Source: CAD feature listing. Evaluate the final solid. Frame: model axes, mm. A direction names the side the tool comes from. Give positions to 0.01 mm unless a question says otherwise; leave off trailing zeros. Write each loop counter-clockwise with the first axis right and the second up, starting at its lowest first coordinate (ties: lowest second). Pieces come first, ordered by that corner, then holes. Notation, with made-up numbers: (49, 42.25) -> (81, 42.25) arc R12 ccw to (81, 57.25) -> close; hole circle Ø2 at (88.25, 20.5). An arc over 180 degrees is marked (long way). Use one line per item in the form item = value. Start each with the question number.
(1) Material intervals for line 1 along Y through (x, z) = (-19.8, 6.3); line 2 along Y through (x, z) = (13, 10.5); line 3 along X through (y, z) = (9, 3), sorted ascending. Write a range as from..to.
(2) Set-up query: faces 1 (the face through (-24, -1, 11.5)), 2 (the face through (-25, 0, 12)), 3 (the face through (-22.5, 0, 13)). Return all of +Z, -Z, +X, -X, +Y, -Y with unobstructed straight access to the full face (end or side cutting, diameter ignored); none if empty.
(3) First-contact query: P1, Ø0.8, axis at x = -23.5, z = 7, coming from the +Y side (3 decimals); P2, Ø1.8, axis at x = 19.8, y = -14.3, coming from the +Z side; P3, Ø1, axis at y = 2, z = 7, coming from the -X side. Flat tips, straight axial feed; report the tip coordinate or a pass-through.
(4) Cut plane D-D, the plane z = 18.75. Output: boundary loops of the cut face in (x, y), and give its area (3 significant figures).
(5) Cut plane C-C, the plane x = -5. Output: boundary loops of the cut face in (y, z), and give its area (4 significant figures).
(6) Cut plane B-B, the plane y = -1. Output: boundary loops of the cut face in (x, z).
(7) Cut plane A-A, the plane z = 6.5. Count the separate pieces of the cut face and the enclosed holes in it, and give its area (3 significant figures).
(8) Draft query along X for faces 4 (the face through (25, 0, 10)), 5 (the face through (24, 10, 10)), 6 (the face through (20.537, 14.976, 4.965)). Return one class per face: pulls with the +X half, pulls with the -X half, needs draft (parallel to the pull), parting line crosses it, or undercut.
from build123d import *

# Parameters (mm, degrees)
F1_DEPTH        = 20
F2_T            = 2.5
F2_T3_DEPTH     = 25
F3_R            = 2.5
F4_DEPTH        = 5
F11_W           = 3
F11_H           = 2
F12_DEPTH       = 5
F13_DEPTH       = 5
F14_W           = 11
F14_H           = 9
F15_DEPTH       = 5
F16_D           = 2
F16_DEPTH       = 10
F16_TIP         = 0.600860619
F17_D           = 2
F17_DEPTH       = 5
F17_TIP         = 0.600860619
F17_ON_F7_D     = 2
F17_ON_F7_DEPTH = 5
F17_ON_F7_TIP   = 0.600860619
F17_ON_F6_D     = 2
F17_ON_F6_DEPTH = 5
F17_ON_F6_TIP   = 0.600860619
F17_ON_F8_D     = 2
F17_ON_F8_DEPTH = 5
F17_ON_F8_TIP   = 0.600860619


# Not quite as in the source:
# - a shell that OpenCascade refuses in one call is made with other operations: the cavity is built on its own and cut out


with BuildPart() as f1:
    # F0 (on Top) → F1 (new body)
    with BuildSketch(Plane.XY):
        with BuildLine():
            Line((-25, 17.5), (-25, 20))
            Line((-25, 20), (-22.5, 20))
            ThreePointArc((-22.5, 20), (-26.767766953, 21.767766953), (-25, 17.5))
        make_face()
        with BuildLine():
            Line((-22.5, 20), (-25, 20))
            Line((-25, 20), (-25, 17.5))
            ThreePointArc((-25, 17.5), (-23.232233047, 18.232233047), (-22.5, 20))
        make_face()
        with BuildLine():
            Line((22.5, 20), (-22.5, 20))
            ThreePointArc((-22.5, 20), (-23.232233047, 18.232233047), (-25, 17.5))
            Line((-25, 17.5), (-25, -17.5))
            ThreePointArc((-25, -17.5), (-23.232233047, -18.232233047), (-22.5, -20))
            Line((-22.5, -20), (22.5, -20))
            ThreePointArc((22.5, -20), (23.232233047, -18.232233047), (25, -17.5))
            Line((25, -17.5), (25, 17.5))
            ThreePointArc((25, 17.5), (23.232233047, 18.232233047), (22.5, 20))
        make_face()
        with BuildLine():
            ThreePointArc((27.5, 20), (25, 22.5), (22.5, 20))
            Line((22.5, 20), (25, 20))
            Line((25, 20), (25, 17.5))
            ThreePointArc((25, 17.5), (26.767766953, 18.232233047), (27.5, 20))
        make_face()
        with BuildLine():
            Line((25, 20), (22.5, 20))
            ThreePointArc((22.5, 20), (23.232233047, 18.232233047), (25, 17.5))
            Line((25, 17.5), (25, 20))
        make_face()
        with BuildLine():
            ThreePointArc((-22.5, -20), (-23.232233047, -18.232233047), (-25, -17.5))
            Line((-25, -17.5), (-25, -20))
            Line((-25, -20), (-22.5, -20))
        make_face()
        with BuildLine():
            Line((-25, -20), (-25, -17.5))
            ThreePointArc((-25, -17.5), (-26.767766953, -21.767766953), (-22.5, -20))
            Line((-22.5, -20), (-25, -20))
        make_face()
        with BuildLine():
            ThreePointArc((27.5, -20), (26.767766953, -18.232233047), (25, -17.5))
            Line((25, -17.5), (25, -20))
            Line((25, -20), (22.5, -20))
            ThreePointArc((22.5, -20), (25, -22.5), (27.5, -20))
        make_face()
        with BuildLine():
            Line((25, -20), (25, -17.5))
            ThreePointArc((25, -17.5), (23.232233047, -18.232233047), (22.5, -20))
            Line((22.5, -20), (25, -20))
        make_face()
    extrude(amount=F1_DEPTH)

    # F2: shell of thickness 2.5, made by hand


with BuildPart() as f2_core1:
    # F2_t2: copy of F1
    add(f1.part)

    # the walls: a layer under each face that stays
    f2_faces = [f2_core1.faces().sort_by_distance(p)[0] for p in [
        (-25, 0, 10),
        (0, -20, 10),
        (25, 0, 10),
        (0, 20, 10),
        (0, 0, 0),
    ]]
    thicken(f2_faces, amount=-F2_T, mode=Mode.SUBTRACT)

    # F2_s4 → F2_t3 (cut)
    with BuildSketch(Plane.XY.offset(-2.5)):
        Polygon((-22.475, 20.025), (-25, 20), (-25, 17.5), (-22.5, 17.5), align=None)
        Polygon((-25.025, 17.475), (-25, 20), (-22.5, 20), (-22.5, 17.5), align=None)
        Polygon((-25.025, -17.475), (-22.5, -17.5), (-22.5, -20), (-25, -20), align=None)
        Polygon((-22.475, -20.025), (-25, -20), (-25, -17.5), (-22.5, -17.5), align=None)
        Polygon((22.475, -20.025), (22.5, -17.5), (25, -17.5), (25, -20), align=None)
        Polygon((25.025, -17.475), (25, -20), (22.5, -20), (22.5, -17.5), align=None)
        Polygon((25.025, 17.475), (22.5, 17.5), (22.5, 20), (25, 20), align=None)
        Polygon((22.475, 20.025), (25, 20), (25, 17.5), (22.5, 17.5), align=None)
    extrude(amount=F2_T3_DEPTH, mode=Mode.SUBTRACT)


with BuildPart() as f1_1:
    add(f1.part)

    # what is left inside the walls is the cavity
    f2_cavity = [f2_core1.part.solids().sort_by_distance(p)[0] for p in [
        (0, -5.833333, 2.525),
    ]]
    add(f2_cavity, mode=Mode.SUBTRACT)

    # F3 (on face) → F4 (join)
    with BuildSketch(Plane.XY.offset(2.5)):
        with Locations((-19.8, 14.3)):
            Circle(F3_R)
        with Locations((19.8, 14.3)):
            Circle(F3_R)
        with Locations((-19.8, -14.3)):
            Circle(F3_R)
        with Locations((19.8, -14.3)):
            Circle(F3_R)
    extrude(amount=F4_DEPTH)

    # F11 (on face) → F12 (cut)
    with BuildSketch(Plane(origin=(0, 20, 0), x_dir=(-1, 0, 0), z_dir=(0, 1, 0))):
        with Locations((-7.3, 4.5)):
            Rectangle(F11_W, F11_H)
    extrude(amount=-F12_DEPTH, mode=Mode.SUBTRACT)

    # F10 (on face) → F13 (cut)
    with BuildSketch(Plane.YZ.offset(25)):
        with BuildLine():
            Line((10.8, 12.5), (8.3, 12.5))
            ThreePointArc((8.3, 12.5), (7.05, 11.25), (8.3, 10))
            Line((8.3, 10), (10.8, 10))
            ThreePointArc((10.8, 10), (12.05, 11.25), (10.8, 12.5))
        make_face()
    extrude(amount=-F13_DEPTH, mode=Mode.SUBTRACT)

    # F14 (on face) → F15 (cut)
    with BuildSketch(Plane(origin=(-25, 0, 0), x_dir=(0, -1, 0), z_dir=(-1, 0, 0))):
        with Locations((1.2, 7)):
            Rectangle(F14_W, F14_H)
    extrude(amount=-F15_DEPTH, mode=Mode.SUBTRACT)

    # F16
    with Locations(Plane.XY.offset(20)):
        with Locations((-25, 20), (25, 20), (-25, -20), (25, -20)):
            Hole(F16_D / 2, depth=F16_DEPTH)
            with Locations((0, 0, -(F16_DEPTH + F16_TIP / 2))):  # 118° drill point
                Cone(0, F16_D / 2, F16_TIP, mode=Mode.SUBTRACT)

    # F17
    with Locations(Plane.XY.offset(7.5)):
        with Locations((-19.8, 14.3)):
            Hole(F17_D / 2, depth=F17_DEPTH)
            with Locations((0, 0, -(F17_DEPTH + F17_TIP / 2))):  # 118° drill point
                Cone(0, F17_D / 2, F17_TIP, mode=Mode.SUBTRACT)

    # F17 on F7
    with Locations(Plane.XY.offset(7.5)):
        with Locations((19.8, 14.3)):
            Hole(F17_ON_F7_D / 2, depth=F17_ON_F7_DEPTH)
            with Locations((0, 0, -(F17_ON_F7_DEPTH + F17_ON_F7_TIP / 2))):  # 118° drill point
                Cone(0, F17_ON_F7_D / 2, F17_ON_F7_TIP, mode=Mode.SUBTRACT)

    # F17 on F6
    with Locations(Plane.XY.offset(7.5)):
        with Locations((-19.8, -14.3)):
            Hole(F17_ON_F6_D / 2, depth=F17_ON_F6_DEPTH)
            with Locations((0, 0, -(F17_ON_F6_DEPTH + F17_ON_F6_TIP / 2))):  # 118° drill point
                Cone(0, F17_ON_F6_D / 2, F17_ON_F6_TIP, mode=Mode.SUBTRACT)

    # F17 on F8
    with Locations(Plane.XY.offset(7.5)):
        with Locations((19.8, -14.3)):
            Hole(F17_ON_F8_D / 2, depth=F17_ON_F8_DEPTH)
            with Locations((0, 0, -(F17_ON_F8_DEPTH + F17_ON_F8_TIP / 2))):  # 118° drill point
                Cone(0, F17_ON_F8_D / 2, F17_ON_F8_TIP, mode=Mode.SUBTRACT)


solid = f1_1.part
Geometry says:
q1.line_1 = -20..-17.5, -16.8..-15.3, -13.3..-11.8, 11.8..13.3, 15.3..16.8, 17.5..20
q1.line_2 = -20..-17.5, 17.5..20
q1.line_3 = -25..-22.5, 22.5..25
q2.face_1 = -X
q2.face_2 = +Z, -Z, -X
q2.face_3 = +Z
q3.P1 = 22.245
q3.P2 = 2.44
q3.P3 = 22.5
q4.outline = (-25, -17.5) arc R2.5 ccw (long way) to (-22.5, -20) -> (22.5, -20) arc R2.5 ccw (long way) to (25, -17.5) -> (25, 17.5) arc R2.5 ccw (long way) to (22.5, 20) -> (-22.5, 20) arc R2.5 ccw (long way) to (-25, 17.5) -> close; hole circle Ø2 at (-25, -20); hole circle Ø2 at (-25, 20); hole (-22.5, -17.5) -> (22.5, -17.5) -> (22.5, 17.5) -> (-22.5, 17.5) -> close; hole circle Ø2 at (25, -20); hole circle Ø2 at (25, 20)
q4.area = 471 mm^2
q5.outline = (-20, 0) -> (20, 0) -> (20, 20) -> (17.5, 20) -> (17.5, 2.5) -> (-17.5, 2.5) -> (-17.5, 20) -> (-20, 20) -> close
q5.area = 187.5 mm^2
q6.outline = (-25, 0) -> (25, 0) -> (25, 20) -> (22.5, 20) -> (22.5, 2.5) -> (-25, 2.5) -> close; (-25, 11.5) -> (-22.5, 11.5) -> (-22.5, 20) -> (-25, 20) -> close
q7.separate_pieces = 5
q7.enclosed_holes = 4
q7.area = 522 mm^2
q8.face_4 = pulls with the +X half
q8.face_5 = needs draft
q8.face_6 = undercut
